from build123d import *

# Parameters (mm, degrees)
SKETCH2_R                 = 2
BOSS_EXTRUDE1_DEPTH       = 70
BOSS_EXTRUDE2_OUTLINE_R   = 2
BOSS_EXTRUDE2_OUTLINE_R_2 = 38
BOSS_EXTRUDE2_DEPTH       = 5
SKETCH5_R                 = 3.75
CUT_EXTRUDE1_DEPTH        = 89
SKETCH6_R                 = 3.75
CUT_EXTRUDE2_DEPTH        = 101


# Read off the part's stored shape, not the designer's step: Boss-Extrude2
with BuildPart() as part:
    # Sketch2 → Boss-Extrude1 (new body)
    with BuildSketch(Plane(origin=(0, 0, 0), x_dir=(1, 0, 0), z_dir=(0, 1, 0))):
        with BuildLine():
            Line((-40.95316077, -50), (-46.54683923, -50))
            ThreePointArc((-46.54683923, -50), (-48.988592627, -48.988592627), (-50, -46.54683923))
            Line((-50, -46.54683923), (-50, -40.95316077))
            Line((-50, -40.95316077), (-50, 40.95316077))
            Line((-50, 40.95316077), (-50, 46.54683923))
            ThreePointArc((-50, 46.54683923), (-48.988592627, 48.988592627), (-46.54683923, 50))
            Line((-46.54683923, 50), (-40.95316077, 50))
            Line((-40.95316077, 50), (-30, 50))
            Line((-30, 50), (-30, 35))
            Line((-30, 35), (30, 35))
            Line((30, 35), (30, 50))
            Line((30, 50), (40.95316077, 50))
            Line((40.95316077, 50), (46.54683923, 50))
            ThreePointArc((46.54683923, 50), (48.988592627, 48.988592627), (50, 46.54683923))
            Line((50, 46.54683923), (50, 40.95316077))
            Line((50, 40.95316077), (50, -40.95316077))
            Line((50, -40.95316077), (50, -46.54683923))
            ThreePointArc((50, -46.54683923), (48.988592627, -48.988592627), (46.54683923, -50))
            Line((46.54683923, -50), (40.95316077, -50))
            Line((40.95316077, -50), (-40.95316077, -50))
        make_face()
        with Locations(Location((-44, 44, 0), (0, 0, 270))):
            Circle(SKETCH2_R, mode=Mode.SUBTRACT)
        with Locations(Location((44, 44, 0), (0, 0, 270))):
            Circle(SKETCH2_R, mode=Mode.SUBTRACT)
        with Locations(Location((44, -44, 0), (0, 0, 270))):
            Circle(SKETCH2_R, mode=Mode.SUBTRACT)
        with Locations(Location((-44, -44, 0), (0, 0, 270))):
            Circle(SKETCH2_R, mode=Mode.SUBTRACT)
        with BuildLine():
            Line((-48, -37.5), (-40.95316077, -37.5))
            ThreePointArc((-40.95316077, -37.5), (-38.511407373, -38.511407373), (-37.5, -40.95316077))
            Line((-37.5, -40.95316077), (-37.5, -48))
            Line((-37.5, -48), (37.5, -48))
            Line((37.5, -48), (37.5, -40.95316077))
            ThreePointArc((37.5, -40.95316077), (38.511407373, -38.511407373), (40.95316077, -37.5))
            Line((40.95316077, -37.5), (48, -37.5))
            Line((48, -37.5), (48, 37.5))
            Line((48, 37.5), (40.95316077, 37.5))
            ThreePointArc((40.95316077, 37.5), (38.511407373, 38.511407373), (37.5, 40.95316077))
            Line((37.5, 40.95316077), (37.5, 48))
            Line((37.5, 48), (32, 48))
            Line((32, 48), (32, 33))
            Line((32, 33), (-32, 33))
            Line((-32, 33), (-32, 48))
            Line((-32, 48), (-37.5, 48))
            Line((-37.5, 48), (-37.5, 40.95316077))
            ThreePointArc((-37.5, 40.95316077), (-38.511407373, 38.511407373), (-40.95316077, 37.5))
            Line((-40.95316077, 37.5), (-48, 37.5))
            Line((-48, 37.5), (-48, -37.5))
        make_face(mode=Mode.SUBTRACT)
    extrude(amount=BOSS_EXTRUDE1_DEPTH)

    # Boss-Extrude2 outline → Boss-Extrude2 (add)
    with BuildSketch(Plane(origin=(0, 70, 0), x_dir=(1, 0, 0), z_dir=(0, 1, 0))):
        with BuildLine():
            ThreePointArc((-46.54683923, 50), (-48.988592627, 48.988592627), (-50, 46.54683923))
            Line((-50, 46.54683923), (-50, -46.54683923))
            ThreePointArc((-50, -46.54683923), (-48.988592627, -48.988592627), (-46.54683923, -50))
            Line((-46.54683923, -50), (46.54683923, -50))
            ThreePointArc((46.54683923, -50), (48.988592627, -48.988592627), (50, -46.54683923))
            Line((50, -46.54683923), (50, 46.54683923))
            ThreePointArc((50, 46.54683923), (48.988592627, 48.988592627), (46.54683923, 50))
            Line((46.54683923, 50), (30, 50))
            Line((30, 50), (30, 35))
            Line((30, 35), (-30, 35))
            Line((-30, 35), (-30, 50))
            Line((-30, 50), (-46.54683923, 50))
        make_face()
        with Locations((-44, -44)):
            Circle(BOSS_EXTRUDE2_OUTLINE_R, mode=Mode.SUBTRACT)
        with Locations((-35, -35.037384196)):
            Circle(BOSS_EXTRUDE2_OUTLINE_R, mode=Mode.SUBTRACT)
        with Locations((44, -44)):
            Circle(BOSS_EXTRUDE2_OUTLINE_R, mode=Mode.SUBTRACT)
        with Locations((35, -35.037384196)):
            Circle(BOSS_EXTRUDE2_OUTLINE_R, mode=Mode.SUBTRACT)
        with Locations((0, -7)):
            Circle(BOSS_EXTRUDE2_OUTLINE_R_2, mode=Mode.SUBTRACT)
        with Locations((-35, 34.962615804)):
            Circle(BOSS_EXTRUDE2_OUTLINE_R, mode=Mode.SUBTRACT)
        with Locations((-44, 44)):
            Circle(BOSS_EXTRUDE2_OUTLINE_R, mode=Mode.SUBTRACT)
        with Locations((35, 34.962615804)):
            Circle(BOSS_EXTRUDE2_OUTLINE_R, mode=Mode.SUBTRACT)
        with Locations((44, 44)):
            Circle(BOSS_EXTRUDE2_OUTLINE_R, mode=Mode.SUBTRACT)
    extrude(amount=BOSS_EXTRUDE2_DEPTH)

    # Sketch5 → Cut-Extrude1 (cut)
    with BuildSketch(Plane(origin=(0, 0, -35), x_dir=(-1, 0, 0), z_dir=(0, 0, -1))):
        with Locations((-25, 15)):
            Circle(SKETCH5_R)
        with Locations((-15, 15)):
            Circle(SKETCH5_R)
        with Locations((-5, 15)):
            Circle(SKETCH5_R)
        with Locations((5, 15)):
            Circle(SKETCH5_R)
        with Locations((15, 15)):
            Circle(SKETCH5_R)
        with Locations((25, 15)):
            Circle(SKETCH5_R)
        with Locations((-25, 25)):
            Circle(SKETCH5_R)
        with Locations((-5, 25)):
            Circle(SKETCH5_R)
        with Locations((5, 25)):
            Circle(SKETCH5_R)
        with Locations((15, 25)):
            Circle(SKETCH5_R)
        with Locations((25, 25)):
            Circle(SKETCH5_R)
        with Locations((-15, 25)):
            Circle(SKETCH5_R)
    extrude(amount=-CUT_EXTRUDE1_DEPTH, mode=Mode.SUBTRACT)

    # Sketch6 → Cut-Extrude2 (cut)
    with BuildSketch(Plane.ZY.offset(50)):
        with Locations((-24.54683923, 15.00014135)):
            Circle(SKETCH6_R)
        with Locations((10.45316077, 15.000000015)):
            Circle(SKETCH6_R)
        with Locations((10.45316077, 27.000000015)):
            Circle(SKETCH6_R)
        with Locations((-24.54683923, 27.00014135)):
            Circle(SKETCH6_R)
    extrude(amount=-CUT_EXTRUDE2_DEPTH, mode=Mode.SUBTRACT)


solid = part.part
The model under review builds one solid part; all positions refer to its coordinate system, in mm. A direction names the side the tool comes from. Round coordinates to 2 decimals unless told otherwise and drop trailing zeros. Order: outer loops, then holes, each group sorted by start corner. A loop starts at its lowest first (then second) coordinate and runs counter-clockwise, first axis right, second up. Notation, with made-up numbers: (41, -5) -> (72, -5) arc R10 cw to (72, 12) -> close; hole circle Ø6 at (-38.5, 80). An arc over 180 degrees is marked (long way). Use CSV: the item, a comma, the result in double quotes. Start each with the question number.
(1) Consider section D-D on y = 16.5. State how many separate pieces and enclosed holes the cut face has, and give its area (3 significant figures).
(2) Consider section C-C on x = -15. Write out the cut boundary in (y, z), and give its area (3 significant figures).
(3) Mouldability with a two-part tool opening along X and no side actions: class faces 4 (the face through (48.99, 23.34, -25.36)), 5 (the face through (25.81, 21.34, -34.01)), 6 (the face through (35.923, 72.465, 36.812)), 7 (the face through (-49.015, 36.975, 48.962)) as pulls with the +X half, pulls with the -X half, needs draft (parallel to the pull), parting line crosses it, or undercut.
(4) Wall thickness on probe 1 along Y at (x, z) = (-15, 49.15); probe 2 along X at (y, z) = (71, -44); probe 3 along X at (y, z) = (40.5, -44): over which ranges is each line inside the solid? List them lowest first. Write a range as from..to.
(5) Consider section B-B on x = -35. Write out the cut boundary in (y, z).
(6) Insertion check: pin 1 (5 mm diameter, centred on x = -35, z = -34.96, fed in from -Y); pin 2 (1.5 mm diameter, centred on x = 5.5, y = 34, fed in from -Z). Each pin has a flat end and moves straight along its axis. Give the tip position at first contact, or say it passes through.
(7) Consider section A-A on z = -4. Write out the cut boundary in (x, y), and give its area (3 significant figures).
(8) Tool access review of faces 1 (the face through (0, 37, -35)), 2 (the face through (45.763, 36.975, -43.056)), 3 (the face through (-1, 35, 48)): name each direction out of +Z, -Z, +X, -X, +Y, -Y from which nothing blocks a thin tool from reaching the whole face with its end or side.
Responses:
1,separate pieces,"16"
1,enclosed holes,"4"
1,area,"994 mm²"
2,outline,"(0, -35) -> (11.25, -35) -> (11.25, -33) -> (0, -33) -> close; (0, 48) -> (11.25, 48) -> (11.25, 50) -> (0, 50) -> close; (18.75, -35) -> (21.25, -35) -> (21.25, -33) -> (18.75, -33) -> close; (18.75, 48) -> (21.25, 48) -> (21.25, 50) -> (18.75, 50) -> close; (28.75, -35) -> (75, -35) -> (75, -27.91) -> (70, -27.91) -> (70, -33) -> (28.75, -33) -> close; (28.75, 48) -> (70, 48) -> (70, 41.91) -> (75, 41.91) -> (75, 50) -> (28.75, 50) -> close"
2,area,"296 mm²"
3,face 4,"needs draft"
3,face 5,"undercut"
3,face 6,"undercut"
3,face 7,"pulls with the -X half"
4,probe 1,"0..11.25, 18.75..21.25, 28.75..75"
4,probe 2,"-50..-46, -42..-30, 30..42, 46..50"
4,probe 3,"-50..-46, -42..-37.5, -32..-30, 30..32, 37.5..42, 46..50"
5,outline,"(0, -50) -> (75, -50) -> (75, -36.96) -> (70, -36.96) -> (70, -48) -> (0, -48) -> close; (0, 48) -> (70, 48) -> (70, 37.04) -> (75, 37.04) -> (75, 50) -> (0, 50) -> close; (70, -32.96) -> (75, -32.96) -> (75, -7.8) -> (70, -7.8) -> close; (70, 21.8) -> (75, 21.8) -> (75, 33.04) -> (70, 33.04) -> close"
6,pin 1,"y = 70"
6,pin 2,"z = -35"
7,outline,"(-50, 0) -> (-48, 0) -> (-48, 70) -> (-36.37, 70) -> (-36.37, 75) -> (-50, 75) -> close; (36.37, 70) -> (48, 70) -> (48, 0) -> (50, 0) -> (50, 75) -> (36.37, 75) -> close"
7,area,"416 mm²"
8,face 1,"-Z, +Y, -Y"
8,face 2,"+Y, -Y"
8,face 3,"-Y"
